Check sheet for the drawn part. Datum: minimum x, y, z corner. Units: mm. A direction names the side the tool comes from. Coordinates: 2 decimals unless noted, no trailing zeros. Loops run counter-clockwise (first coordinate to the right, second up) from the corner with the lowest first, then second, coordinate; pieces in that order, holes last.
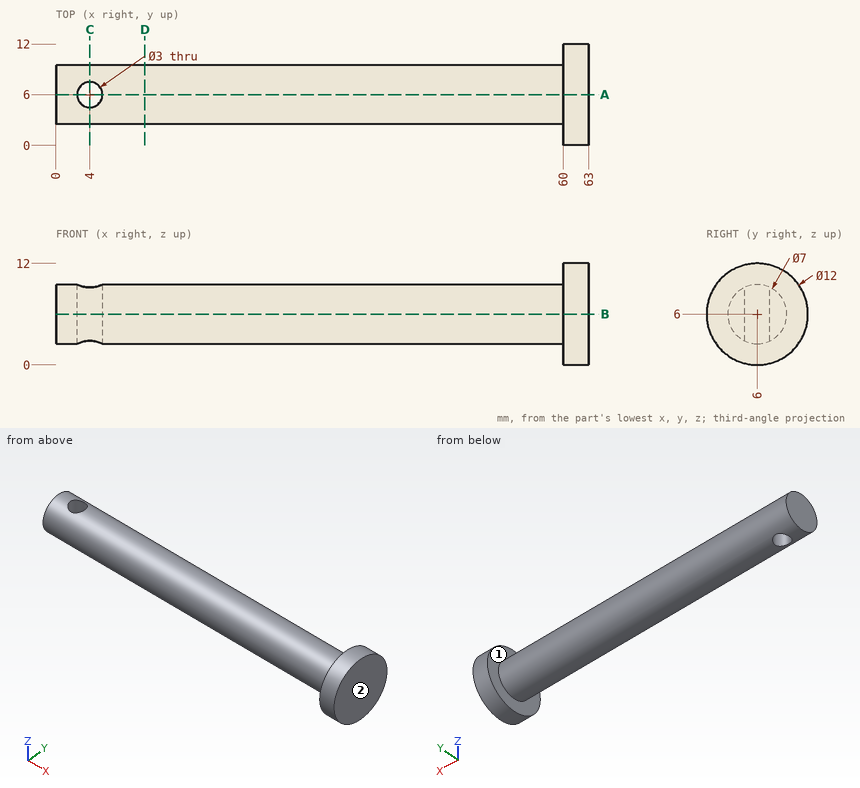
(1) Sectioned sample at A-A on y = 6. Record the cut outline in (x, z).
Findings:
outline: (0, 2.5) - (2.5, 2.5) - (2.5, 9.5) - (0, 9.5) - close; (5.5, 2.5) - (60, 2.5) - (60, 0) - (63, 0) - (63, 12) - (60, 12) - (60, 9.5) - (5.5, 9.5) - close
(2) Sectioned sample at D-D on x = 10.5. Record the cut outline in (y, z), and give its area (3 significant figures).
Findings:
outline: circle Ø7 at (6, 6)
area: 38.5 mm2
(3) Sectioned sample at B-B on z = 6. Record the cut outline in (x, y).
Findings:
outline: (0, 2.5) - (60, 2.5) - (60, 0) - (63, 0) - (63, 12) - (60, 12) - (60, 9.5) - (0, 9.5) - close; hole circle Ø3 at (4, 6)
(4) Scan lines: L1, parallel to X at y = 6, z = 6.25; L2, parallel to X at y = 4.75, z = 9.5; L3, parallel to Y at x = 4, z = 5.75. Record each from-to range of solid material in increasing order.
Findings:
L1: x = 0 to 2.5, 5.5 to 63
L2: x = 60 to 63
L3: y = 2.51 to 4.5, 7.5 to 9.49
(5) Gauge pin test, flat ends, axial feed: pin 1 Ø4 at (x, z) = (47, 9.5) entering from +Y; pin 2 Ø6 at (y, z) = (3.5, 3.5) entering from -X; pin 3 Ø4 at (x, y) = (38.5, 10) entering from +Z; pin 4 Ø1.5 at (x, z) = (11, 7) entering from -Y. Record the tip position at first contact, or that the pin passes through.
Findings:
pin 1: stops at y = 9.16
pin 2: stops at x = 0
pin 3: stops at z = 8.87
pin 4: stops at y = 2.51
(6) Sectioned sample at C-C on x = 4. Record the cut outline in (y, z), and give its area (3 significant figures).
Findings:
outline: (4.5, 2.84) - (4.5, 9.16) arc R3.5 ccw to start; (7.5, 2.84) arc R3.5 ccw to (7.5, 9.16) - close
area: 18.1 mm2
(7) Access from +Z, -Z, +X, -X, +Y, -Y to the whole of each face (thin tool, end or side, straight path). Record for the marked faces 1 and 2.
Findings:
face 1: -X
face 2: +Z, -Z, +X, +Y, -Y
